Could you check a few things on this model? Use its own coordinates, in mm. Round coordinates to 2 decimals unless told otherwise and drop trailing zeros. Write each loop counter-clockwise with the first axis right and the second up, starting at its lowest first coordinate (ties: lowest second). Pieces come first, ordered by that corner, then holes. Notation, with made-up numbers: (-15.75, -21.5) -> (18.25, -21.5) arc R14 cw to (18.25, -13.5) -> close; hole circle Ø2 at (16.5, -32). An arc over 180 degrees is marked (long way). Return JSON: item names as keys, results as strings.
Autodesk Inventor part; units mm, degrees
ref_plane "YZ Plane" through (0, 0, 0) normal (1, 0, 0) x (0, 1, 0)
ref_plane "XZ Plane" through (0, 0, 0) normal (0, 1, 0) x (-1, 0, 0)
ref_plane "XY Plane" through (0, 0, 0) normal (0, 0, 1) x (1, 0, 0)
sketch "Sketch1" plane through (0, 0, 0) normal (0, 1, 0) x (-1, 0, 0)
  line L0 (0, 0) -> (0, -2.75)
  line L1 (0, 0) -> (9.5, 0)
  line L2 (9.5, 0) -> (9.5, -1.5)
  line L3 (9.5, -1.5) -> (2, -1.5)
  line L4 (2, -1.5) -> (0.75, -2.75)
  line L5 (2, -1.5) -> (3.7678, -1.5) construction
  line L6 (0.75, -2.75) -> (0, -2.75)
  dimension "d0" = 2.75
  dimension "d1" = 9.5
  dimension "d2" = 1.5
  dimension "d3" = 7.5
  dimension "d4" = 135
revolve "Revolution1" add sketch "Sketch1" angle 360 about axis through (0, 0, 0) along (-1, 0, 0)
fillet "Fillet1" radius 0.25 2 edges at (-0.75, 0, 2.75) (0, 0, 2.75)
sketch "Sketch2" plane through (0, 0, 0) normal (1, 0, 0) x (0, 0, -1)
  line L0 (-1.5, 0.5) -> (1.5, 0.5)
  line L1 (1.5, 0.5) -> (1.5, -0.5)
  line L2 (1.5, -0.5) -> (-1.5, -0.5)
  line L3 (-1.5, -0.5) -> (-1.5, 0.5)
  line L4 (-1.5, 0.5) -> (1.5, -0.5) construction
  line L5 (1.5, 0.5) -> (-1.5, -0.5) construction
  line L6 (0.5, 1.5) -> (-0.5, 1.5)
  line L7 (-0.5, 1.5) -> (-0.5, -1.5)
  line L8 (-0.5, -1.5) -> (0.5, -1.5)
  line L9 (0.5, -1.5) -> (0.5, 1.5)
  line L10 (0.5, 1.5) -> (-0.5, -1.5) construction
  line L11 (-0.5, 1.5) -> (0.5, -1.5) construction
  point P0 (0, 0)
  point P1 (0.5, 0.5)
  point P2 (-0.5, 0.5)
  point P3 (-0.5, -0.5)
  point P4 (0.5, -0.5)
  dimension "d9" = 3
  dimension "d10" = 1
  dimension "d11" = 1
  dimension "d12" = 3
extrude "Extrusion1" cut sketch "Sketch2" against normal blind 1.5
sketch "Sketch3" plane through (-9.5, 0, 0) normal (-1, 0, 0) x (0, 0, 1)
  circle A0 centre (0, 0) radius 1.5
extrude "Extrusion2" add sketch "Sketch3" along normal blind 10.5
thread "Thread2"
chamfer "Chamfer2" distance 0.25 angle 45 1 edges at (-20, 0, -1.5)
sketch "Sketch4" plane through (-20, 0, 0) normal (-1, 0, 0) x (0, 0, 1)
  circle A0 centre (0, 0) radius 1.5
extrude "Extrusion3" add sketch "Sketch4" along normal blind 10 and the other way blind 5
chamfer "Chamfer3" distance 0.25 angle 45 1 edges at (-30, 0, -1.5)
properties part number "M3_Long_Bolt" material "Steel, Alloy"
1) Will these pins go through, and if not, where does the flat tip stop? pin 1 Ø2 at (y, z) = (0, -1) entering from +X; pin 2 Ø1 at (x, y) = (-4, 0.5) entering from +Z; pin 3 Ø1 at (x, y) = (-16, -0.5) entering from -Z; pin 4 Ø1.1 at (x, z) = (-0.5, 1) entering from +Y.
Return value:
{"pin 1": "x = 0", "pin 2": "z = 1.5", "pin 3": "z = -1.5", "pin 4": "y = 2.71"}
2) I want a section at A-A, the plane x = -9. Please give me the cut outline in (y, z).
Return value:
{"outline": "circle Ø3 at (0, 0)"}
3) Thinking about a two-plate mould opening in Z: for faces 1 (the face through (-30, 0, 0)), 2 (the face through (-0.445, 2.727, 0.358)), 3 (the face through (-1, -0.5, 1)), which applies, pulls with the +Z half, pulls with the -Z half, needs draft (parallel to the pull), parting line crosses it, or undercut?
Return value:
{"face 1": "needs draft", "face 2": "parting line crosses it", "face 3": "undercut"}
4) If I drill on probe 1 along Y at (x, z) = (-1.25, 0.3); probe 2 along Y at (x, z) = (-6.75, 0.1); probe 3 along X at (y, z) = (0.1, -0.4), over which ranges is the centre line in solid material (lowest first)? Write a range as [from, to].
Return value:
{"probe 1": "[-2.23, -1.5], [1.5, 2.23]", "probe 2": "[-1.5, 1.5]", "probe 3": "[-30, -1.5]"}
